Can you work these out from the model? Positions are in its coordinate system, mm. Face numbers are marked on the shaded views. A direction names the side the tool comes from. Round coordinates to 2 decimals unless told otherwise and drop trailing zeros. Order: outer loops, then holes, each group sorted by start corner. A loop starts at its lowest first (then second) coordinate and runs counter-clockwise, first axis right, second up. Notation, with made-up numbers: (69.5, 0) -> (121.5, 0) arc R20 ccw to (121.5, 12) -> close; hole circle Ø11 at (-38.5, 16.25). An arc over 180 degrees is marked (long way). One line per item, written item: value.
```python
from build123d import *

# Parameters (mm, degrees)
SCHIZZO1_W                   = 16.52
SCHIZZO1_H                   = 8.52
SCHIZZO1_W_2                 = 14
SCHIZZO1_H_2                 = 6
ESTRUSIONE_SOTTILE1_DEPTH    = 20
SCHIZZO2_W                   = 16.52
SCHIZZO2_H                   = 8.52
ESTRUSIONE_ESTRUSIONE1_DEPTH = 1.5
RACCORDO1_R                  = 1.6
RACCORDO2_R                  = 0.5


with BuildPart() as part:
    # Schizzo1 → Estrusione-Sottile1 (new body)
    with BuildSketch(Plane.XY):
        Rectangle(SCHIZZO1_W, SCHIZZO1_H)
        Rectangle(SCHIZZO1_W_2, SCHIZZO1_H_2, mode=Mode.SUBTRACT)
    extrude(amount=ESTRUSIONE_SOTTILE1_DEPTH)

    # Schizzo2 → Estrusione-Estrusione1 (add)
    with BuildSketch(Plane.XY.offset(20)):
        Rectangle(SCHIZZO2_W, SCHIZZO2_H)
    extrude(amount=ESTRUSIONE_ESTRUSIONE1_DEPTH)

    # Raccordo1
    raccordo1_edges = [part.edges().sort_by_distance(p)[0] for p in [
        (0, -4.26, 21.5),
        (8.26, 0, 21.5),
        (0, 4.26, 21.5),
        (-8.26, 0, 21.5),
        (-8.26, 4.26, 10.75),
        (8.26, 4.26, 10.75),
        (8.26, -4.26, 10.75),
        (-8.26, -4.26, 10.75),
    ]]
    fillet(raccordo1_edges, radius=RACCORDO1_R)

    # Raccordo2
    raccordo2_edges = [part.edges().sort_by_distance(p)[0] for p in [
        (-7, 3, 10),
        (-7, -3, 10),
        (7, -3, 10),
        (7, 3, 10),
        (-7, 0, 20),
        (0, -3, 20),
        (7, 0, 20),
        (0, 3, 20),
    ]]
    fillet(raccordo2_edges, radius=RACCORDO2_R)


solid = part.part
```
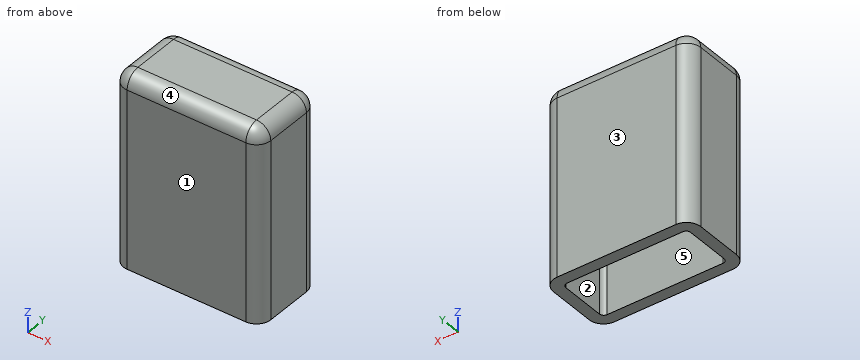
Q1. Will these pins go through, and if not, where does the flat tip stop? pin 1 Ø1 at (y, z) = (-3, 10.5) entering from -X; pin 2 Ø4 at (x, y) = (2.5, -0.5) entering from -Z.
Answers below:
pin 1: x = -8.26
pin 2: z = 20
Q2. We'd pull the mould along Y, two halves only. Please class the marked faces 3, 4 and 5: released by +Y, released by -Y, zero draft, split by the parting line, or undercut.
Answers below:
face 3: released by +Y
face 4: released by -Y
face 5: undercut
Q3. Please list where these lines run through material, in increasing order: line 1 along X through (y, z) = (-2.5, 7); line 2 along Y through (x, z) = (0.5, 7.5); line 3 along Z through (x, y) = (6, 1.75).
Answers below:
line 1: -8.26 to -7, 7 to 8.26
line 2: -4.26 to -3, 3 to 4.26
line 3: 20 to 21.5
Q4. I want a section at A-A on z = 15.5. List the corners of the cut face in (x, y) for me.
Answers below:
outline: (-8.26, -2.66) arc R1.6 ccw to (-6.66, -4.26) -> (6.66, -4.26) arc R1.6 ccw to (8.26, -2.66) -> (8.26, 2.66) arc R1.6 ccw to (6.66, 4.26) -> (-6.66, 4.26) arc R1.6 ccw to (-8.26, 2.66) -> close; hole (-7, -2.5) arc R0.5 ccw to (-6.5, -3) -> (6.5, -3) arc R0.5 ccw to (7, -2.5) -> (7, 2.5) arc R0.5 ccw to (6.5, 3) -> (-6.5, 3) arc R0.5 ccw to (-7, 2.5) -> close
Q5. I want a section at B-B on x = -4.75. List the corners of the cut face in (y, z) for me, plus the area to 3 significant figures.
Answers below:
outline: (-4.26, 0) -> (-3, 0) -> (-3, 19.5) arc R0.5 cw to (-2.5, 20) -> (2.5, 20) arc R0.5 cw to (3, 19.5) -> (3, 0) -> (4.26, 0) -> (4.26, 19.9) arc R1.6 ccw to (2.66, 21.5) -> (-2.66, 21.5) arc R1.6 ccw to (-4.26, 19.9) -> close
area: 62.2 mm^2
Q6. On a 3-axis mill with a long thin cutter (end or side, diameter ignored), from which of +Z, -Z, +X, -X, +Y, -Y can I reach the whole of each face in a straight line? I mean the marked faces 1 and 2. Say none if no direction works.
Answers below:
face 1: +Z, -Z, +X, -X, -Y
face 2: -Z
Q7. I want a section at C-C on y = 0.5. List the corners of the cut face in (x, z) for me, plus the area to 3 significant figures.
Answers below:
outline: (-8.26, 0) -> (-7, 0) -> (-7, 19.5) arc R0.5 cw to (-6.5, 20) -> (6.5, 20) arc R0.5 cw to (7, 19.5) -> (7, 0) -> (8.26, 0) -> (8.26, 19.9) arc R1.6 ccw to (6.66, 21.5) -> (-6.66, 21.5) arc R1.6 ccw to (-8.26, 19.9) -> close
area: 74.2 mm^2
Q8. I want a section at D-D on y = 3.5. List the corners of the cut face in (x, z) for me, plus the area to 3 significant figures.
Answers below:
outline: (-8.02, 0) -> (8.02, 0) -> (8.02, 19.9) arc R1.36 ccw to (6.66, 21.26) -> (-6.66, 21.26) arc R1.36 ccw to (-8.02, 19.9) -> close
area: 340 mm^2
